from build123d import *

# Parameters (mm, degrees)
SKETCH2_R           = 3.5
BOSS_EXTRUDE1_DEPTH = 10
SKETCH3_R           = 1.5
CUT_EXTRUDE1_DEPTH  = 10
CHAMFER1_SIZE       = 0.2
CHAMFER2_SIZE       = 0.1


with BuildPart() as part:
    # Sketch2 → Boss-Extrude1 (new body)
    with BuildSketch(Plane.XY):
        with Locations((6.092427376, -11.118651223)):
            Circle(SKETCH2_R)
    extrude(amount=BOSS_EXTRUDE1_DEPTH)

    # Sketch3 → Cut-Extrude1 (cut)
    with BuildSketch(Plane.XY.offset(10)):
        with Locations((6.092427376, -11.118651223)):
            Circle(SKETCH3_R)
    extrude(amount=-CUT_EXTRUDE1_DEPTH, mode=Mode.SUBTRACT)

    # Chamfer1
    chamfer1_edges = [part.edges().sort_by_distance(p)[0] for p in [
        (2.592427376, -11.118651223, 0),
        (2.592427376, -11.118651223, 10),
    ]]
    chamfer(chamfer1_edges, length=CHAMFER1_SIZE)

    # Chamfer2
    chamfer2_edges = [part.edges().sort_by_distance(p)[0] for p in [
        (4.592427376, -11.118651223, 0),
        (4.592427376, -11.118651223, 10),
    ]]
    chamfer(chamfer2_edges, length=CHAMFER2_SIZE)


solid = part.part
Check sheet for the modelled part. Datum: model origin and axes. Units: mm. Give positions to 0.01 mm unless a question says otherwise; leave off trailing zeros. Loops run counter-clockwise (first coordinate to the right, second up) from the corner with the lowest first, then second, coordinate; pieces in that order, holes last. Notation, with made-up numbers: M -27,76.25 L 0,76.25 A32 cw 0,107.25 Z; hole C -2.5,76.5 d5. An arc over 180 degrees is marked long. Use a Markdown table: item, result. Add a question column.
Q1. Mould release check, pull along Y, two halves, no side actions. Record for faces 1 (the flat face through (5, -13, 10)), 2 (the cylindrical face through (7.48, -11.69, 5.07)), 3 (the cylindrical face through (5.334, -14.535, 4.933)): pulls with the +Y half, pulls with the -Y half, needs draft (parallel to the pull), parting line crosses it, or undercut.
Q2. Sectioned sample at A-A, the plane z = 9.25. Record the cut outline in (x, y).
Q3. Scan lines: line 1 along X through (y, z) = (-11.25, 0.75); line 2 along X through (y, z) = (-12, 4); line 3 along Y through (x, z) = (6.5, 5.5). Record each from-to range of solid material in increasing order. Write a range as [from, to].
Q4. Go/stop test with flat-tipped pins: pin 1 (1.5 mm diameter, centred on y = -13, z = 5.5, fed in from -X); pin 2 (1.5 mm diameter, centred on x = 8.5, z = 2.5, fed in from -Y). Record where each tip stops, or that it passes through.
Verdict:
| question | item | result |
|---|---|---|
| 1 | face 1 | needs draft |
| 1 | face 2 | undercut |
| 1 | face 3 | parting line crosses it |
| 2 | outline | C 6.09,-11.12 d7; hole C 6.09,-11.12 d3 |
| 3 | line 1 | [2.59, 4.6], [7.59, 9.59] |
| 3 | line 2 | [2.71, 4.88], [7.31, 9.48] |
| 3 | line 3 | [-14.59, -12.56], [-9.68, -7.64] |
| 4 | pin 1 | x = 2.78 |
| 4 | pin 2 | y = -14.2 |
